Study the drawing (mm; zero at the part's minimum x, y, z) and answer. A direction names the side the tool comes from. Round coordinates to 2 decimals unless told otherwise and drop trailing zeros. Write each loop counter-clockwise with the first axis right and the second up, starting at its lowest first coordinate (ties: lowest second). Pieces come first, ordered by that corner, then holes. Notation, with made-up numbers: (-5.5, -5.5) - (41.5, -5.5) arc R15 ccw to (41.5, 0.5) - close; hole circle Ø3 at (49, 60.5). An arc over 180 degrees is marked (long way). Return JSON: item names as keys, results as strings. Group by question number.
(1) Which of the six approach directions +Z, -Z, +X, -X, +Y, -Y give full straight-line access (tool end or side, diameter ignored) to the marked faces 1 and 2?
(2) Section B-B, the plane x = 15 is taken. Write down the section's boundary in (y, z).
(3) Each of these flat-tipped pins is pushed along its axis until it touches: pin 1 (19 mm diameter, centred on x = 16, z = 29.5, fed in from -Y); pin 2 (1.5 mm diameter, centred on x = 5.5, y = 9.5, fed in from +Z). Where does it stop, or does it pass through?
(4) Find the intervals of material crossed by line 1 along X through (y, z) = (57.5, 29.21); line 2 along Z through (x, y) = (25, 53); line 3 along Y through (x, z) = (6, 28.5), in increasing order. Write a range as [from, to].
(5) Section A-A, the plane x = 29 is taken. Write down the section's boundary in (y, z), then the cut area to 3 significant figures.
(6) Section C-C, the plane z = 46.5 is taken. Write down the section's boundary in (x, y).
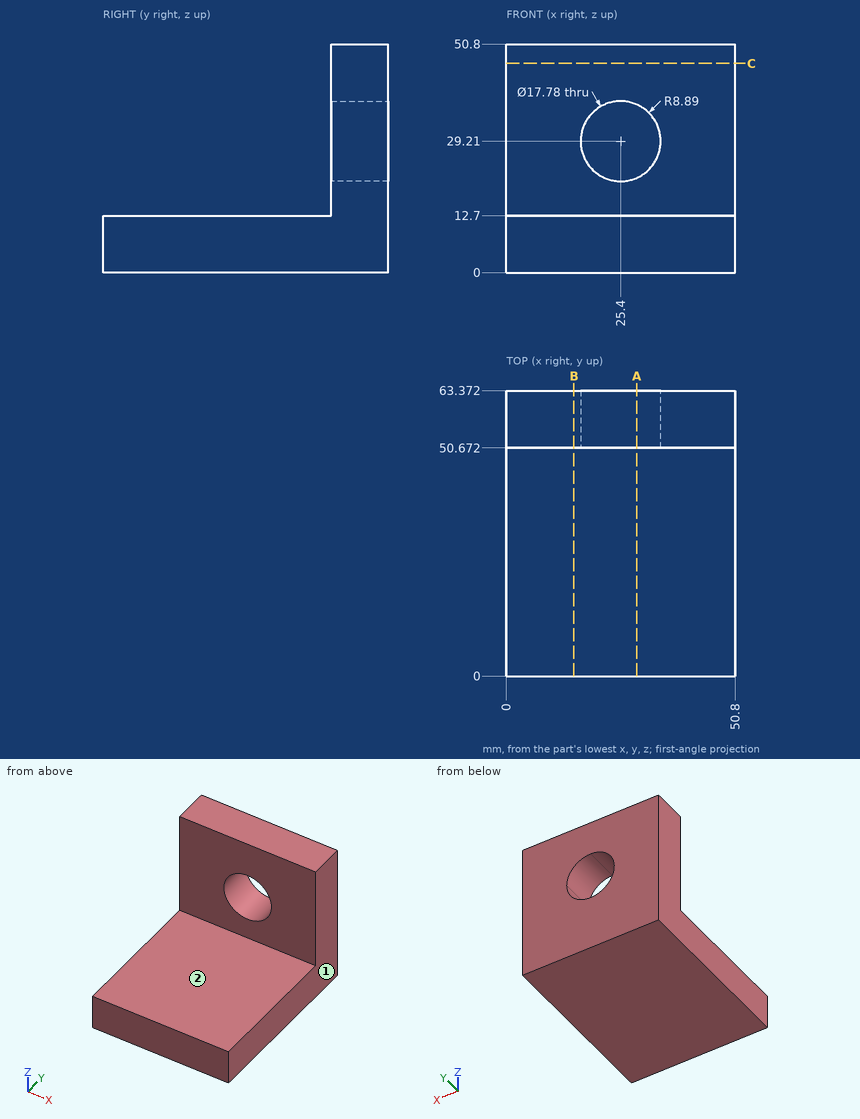
Working result:
{
 "1": {"face 1": "+Z, -Z, +X, +Y, -Y", "face 2": "+Z, +X, -X, -Y"},
 "2": {"outline": "(0, 0) - (63.37, 0) - (63.37, 50.8) - (50.67, 50.8) - (50.67, 12.7) - (0, 12.7) - close"},
 "3": {"pin 1": "stops at y = 50.67", "pin 2": "stops at z = 12.7"},
 "4": {"line 1": "x = [0, 16.51], [34.29, 50.8]", "line 2": "z = [0, 20.33], [38.09, 50.8]", "line 3": "y = [50.67, 63.37]"},
 "5": {"outline": "(0, 0) - (63.37, 0) - (63.37, 21.08) - (50.67, 21.08) - (50.67, 12.7) - (0, 12.7) - close; (50.67, 37.34) - (63.37, 37.34) - (63.37, 50.8) - (50.67, 50.8) - close", "area": "1,080 mm^2"},
 "6": {"outline": "(0, 50.67) - (50.8, 50.67) - (50.8, 63.37) - (0, 63.37) - close"}
}
